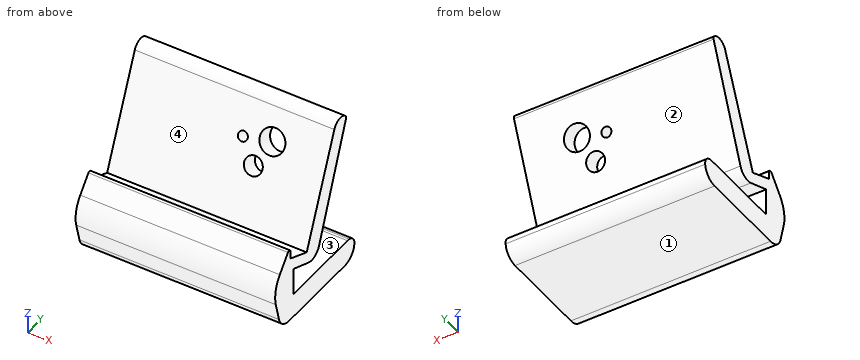
```python
from build123d import *

# Parameters (mm, degrees)
F1_DEPTH     = 61
F2_R         = 9.670635699
F3_R         = 0.6712415125
F4_R         = 3.1919162273
F5_R         = 4.5432418233
F6_R         = 5
F7_R         = 3.8651714317
F7_R_2       = 1.4867583823
F7_R_3       = 2.8155117611
F8_DEPTH     = 25
F10_DEPTH    = 75.5
F11_R        = 3.8627416998
F12_T1_DEPTH = 73.5452662192
F13_R        = 3
F14_R        = 1


# Not quite as in the source:
# - a fillet or chamfer that OpenCascade refuses, or shapes differently, is made with other operations: its cross-section is extruded or revolved along the edge and cut away or added


with BuildPart() as f1:
    # F0 (on Right) → F1 (new body)
    with BuildSketch(Plane.YZ):
        with BuildLine():
            add(Edge.make_bspline(
                [(18.1424543803, -35.0754142348), (0, -24.5931053673), (21.0989990325, 0), (4.9723746061, 18.9487867674)],
                knots=[0, 0, 0, 0, 55.6063422209, 55.6063422209, 55.6063422209, 55.6063422209], degree=3))
            Line((4.9723746061, 18.9487867674), (-10.6166982745, -18.1424543803))
            Line((-10.6166982745, -18.1424543803), (-18.4527349874, -14.8490475373))
            Line((-18.4527349874, -14.8490475373), (-18.4527349874, -10.6166952334))
            Line((-18.4527349874, -10.6166952334), (-26.7433237145, -20.5614495141))
            Line((-26.7433237145, -20.5614495141), (-22.9804446479, -35.0754142348))
            Line((-22.9804446479, -35.0754142348), (18.1424543803, -35.0754142348))
        make_face()
    extrude(amount=F1_DEPTH)

    # F2
    f2_edges = [f1.edges().sort_by_distance(p)[0] for p in [
        (30.5, -26.743324, -20.56145),
    ]]
    fillet(f2_edges, radius=F2_R)

    # F3
    f3_edges = [f1.edges().sort_by_distance(p)[0] for p in [
        (30.5, -18.452735, -10.616695),
    ]]
    fillet(f3_edges, radius=F3_R)

    # F4
    f4_edges = [f1.edges().sort_by_distance(p)[0] for p in [
        (30.5, 4.972375, 18.948787),
    ]]
    fillet(f4_edges, radius=F4_R)

    # F5
    f5_edges = [f1.edges().sort_by_distance(p)[0] for p in [
        (30.5, 18.142454, -35.075414),
    ]]
    fillet(f5_edges, radius=F5_R)

    # F6
    f6_edges = [f1.edges().sort_by_distance(p)[0] for p in [
        (30.5, -22.980445, -35.075414),
    ]]
    fillet(f6_edges, radius=F6_R)

    # F7 (on face) → F8 (cut)
    with BuildSketch(Plane(origin=(0, -2.542493383, 1.0685842107), x_dir=(1, 0, 0), z_dir=(0, -0.9218866721, 0.3874596286))):
        with Locations((44.390194118, 4.044146277)):
            Circle(F7_R)
        with Locations((35.7474051416, 2.4390574545)):
            Circle(F7_R_2)
        with Locations((40.5626744032, -4.1047660634)):
            Circle(F7_R_3)
    extrude(amount=-F8_DEPTH, mode=Mode.SUBTRACT)

    # F9 (on face) → F10 (cut)
    with BuildSketch(Plane.YZ.offset(61)):
        Polygon((17.7633237159, 10.0974902644), (8.4745825412, 13.7160523356), (-6.0518267564, -23.5728081316), (-17.0180739519, -19.3007495805), (-17.0180739519, -27.6472643018), (21.4816201478, -27.6472643018), align=None)
    extrude(amount=-F10_DEPTH, mode=Mode.SUBTRACT)

    # F11
    f11_edges = [f1.edges().sort_by_distance(p)[0] for p in [
        (30.5, -6.051827, -23.572808),
    ]]
    fillet(f11_edges, radius=F11_R)

    # F12: fillet of radius 5 on 1 edges, made by hand

    # F12_s2 → F12_t1 (cut)
    with BuildSketch(Plane.YZ.offset(-6.2726331096)):
        with BuildLine():
            ThreePointArc((8.9937485165, -27.6472643018), (10.5238649897, -27.8871441795), (11.9071638019, -28.5837668704))
            Line((11.9071638019, -28.5837668704), (11.9654321077, -28.5024969218))
            ThreePointArc((11.9654321077, -28.5024969218), (11.7885278554, -28.0794589932), (11.5959390896, -27.6108577379))
            Line((11.5959390896, -27.6108577379), (11.5028017603, -27.5472643018))
            Line((11.5028017603, -27.5472643018), (8.9937485165, -27.5472643018))
            Line((8.9937485165, -27.5472643018), (8.9937485165, -27.6472643018))
        make_face()
    extrude(amount=F12_T1_DEPTH, mode=Mode.SUBTRACT)

    # F13
    f13_edges = [f1.edges().sort_by_distance(p)[0] for p in [
        (30.5, 11.907164, -28.583767),
    ]]
    fillet(f13_edges, radius=F13_R)

    # F14
    f14_edges = [f1.edges().sort_by_distance(p)[0] for p in [
        (30.5, 8.474583, 13.716052),
    ]]
    fillet(f14_edges, radius=F14_R)


solid = f1.part
```
Check sheet for the modelled part. Datum: model origin and axes. Units: mm. Face numbers are marked on the shaded views. Give positions to 0.01 mm unless a question says otherwise; leave off trailing zeros. Write each loop counter-clockwise with the first axis right and the second up, starting at its lowest first coordinate (ties: lowest second). Pieces come first, ordered by that corner, then holes. Notation, with made-up numbers: (65, 35.5) -> (86, 35.5) arc R14 ccw to (86, 43.5) -> close; hole circle Ø11 at (53.25, -23.75). An arc over 180 degrees is marked (long way). Use CSV: the item, a comma, the result in double quotes. Start each with the question number.
Q1. Scan lines: line 1 along Z through (x, y) = (13, -11); line 2 along Z through (x, y) = (45, -14.5); line 3 along Y through (x, z) = (4.5, -12). Record each from-to range of solid material in increasing order.
Q2. Cross-section at C-C on z = -8.5. Enter the section's corners in (x, y).
Q3. Cross-section at B-B on y = -12. Enter the section's corners in (x, z).
Q4. Cross-section at D-D on y = -21. Enter the section's corners in (x, z), and give its area (3 significant figures).
Q5. Depth check by flat-ended pin: P1, Ø8, axis at y = -7.5, z = 0, coming from the -X side; P2, Ø8, axis at y = -14, z = -26.5, coming from the -X side; P3, Ø21, axis at x = 35.5, y = -5.5, coming from the +Z side; P4, Ø2, axis at x = 45, z = -17.5, coming from the -Y side. Enter the tip coordinate at first touch or a pass-through.
Q6. Release check for a two-part mould opening along Z. For the marked faces 1, 2, 3 and 4 record: +Z half, -Z half, draft (parallel to the pull), parting line (faces both ways), or undercut.
Q7. Cross-section at A-A on y = -6. Enter the section's corners in (x, z), and give its area (3 significant figures).
Working result:
1,line 1,"z = -35.08 to -27.65, -21.65 to -17.98"
1,line 2,"z = -35.08 to -27.65, -20.28 to -16.51"
1,line 3,"y = -19.6 to -18.64, -8.04 to -1.54"
2,outline,"(0, -6.56) -> (61, -6.56) -> (61, -0.18) -> (0, -0.18) -> close"
3,outline,"(0, -35.08) -> (61, -35.08) -> (61, -27.65) -> (0, -27.65) -> close; (0, -21.26) -> (61, -21.26) -> (61, -17.56) -> (0, -17.56) -> close"
4,outline,"(0, -34.71) -> (61, -34.71) -> (61, -13.67) -> (0, -13.67) -> close"
4,area,"1,280 mm^2"
5,P1,"passes through"
5,P2,"stops at x = 0"
5,P3,"stops at z = 15.4"
5,P4,"stops at y = -24.73"
6,face 1,"-Z half"
6,face 2,"undercut"
6,face 3,"undercut"
6,face 4,"+Z half"
7,outline,"(0, -35.08) -> (61, -35.08) -> (61, -27.65) -> (0, -27.65) -> close; (0, -21.71) -> (61, -21.71) -> (61, -7.16) -> (0, -7.16) -> close"
7,area,"1,340 mm^2"
